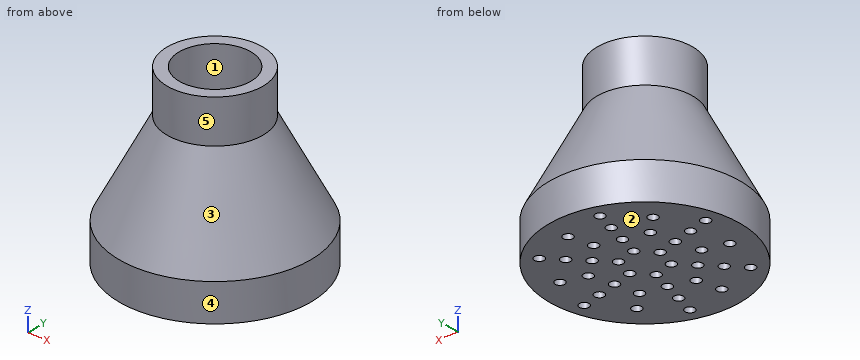
```python
from build123d import *

# Parameters (mm, degrees)
F0_R     = 25.4
F1_DEPTH = 31.75
F4_T     = -2.54
F5_R     = 12.7
F5_R_2   = 9.525
F6_DEPTH = 11.43
F7_R     = 25.4
F7_R_2   = 1.27
F8_DEPTH = 2.54


with BuildPart() as f1:
    # F0 (on Top) → F1 (new body)
    with BuildSketch(Plane.XY):
        Circle(F0_R)
    extrude(amount=F1_DEPTH)

    # F2 (on Right) → F3 (revolve, cut)
    with BuildSketch(Plane.YZ):
        Polygon((-29.21, 31.75), (-29.21, 0), (-12.7, 31.75), align=None)
    revolve(axis=Axis((0, 0, 15.875), (0, 0, -1)), mode=Mode.SUBTRACT)

    # F4
    f4_openings = [f1.faces().sort_by_distance(p)[0] for p in [
        (0, 0, 0),
        (0, 0, 31.75),
    ]]
    offset(amount=F4_T, openings=f4_openings)

    # F5 (on face) → F6 (join)
    with BuildSketch(Plane.XY.offset(31.75)):
        Circle(F5_R)
        Circle(F5_R_2, mode=Mode.SUBTRACT)
    extrude(amount=F6_DEPTH)

    # F7 (on face) → F8 (join)
    with BuildSketch(Plane(origin=(0, 0, 0), x_dir=(1, 0, 0), z_dir=(0, 0, -1))):
        Circle(F7_R)
        with Locations((-13.470384, -13.470384)):
            Circle(F7_R_2, mode=Mode.SUBTRACT)
        with Locations((-5.578226, -20.818224)):
            Circle(F7_R_2, mode=Mode.SUBTRACT)
        with Locations((-4.18367, -15.613668)):
            Circle(F7_R_2, mode=Mode.SUBTRACT)
        with Locations((-20.818224, -5.578226)):
            Circle(F7_R_2, mode=Mode.SUBTRACT)
        with Locations((-15.613668, -4.18367)):
            Circle(F7_R_2, mode=Mode.SUBTRACT)
        with Locations((-8.980256, -8.980256)):
            Circle(F7_R_2, mode=Mode.SUBTRACT)
        with Locations((-2.789113, -10.409112)):
            Circle(F7_R_2, mode=Mode.SUBTRACT)
        with Locations((-10.409112, -2.789113)):
            Circle(F7_R_2, mode=Mode.SUBTRACT)
        with Locations((-1.394557, -5.204557)):
            Circle(F7_R_2, mode=Mode.SUBTRACT)
        with Locations((-5.204557, -1.394557)):
            Circle(F7_R_2, mode=Mode.SUBTRACT)
        with Locations((4.930503, -18.400887)):
            Circle(F7_R_2, mode=Mode.SUBTRACT)
        with Locations((15.239998, -15.239998)):
            Circle(F7_R_2, mode=Mode.SUBTRACT)
        with Locations((3.287002, -12.267258)):
            Circle(F7_R_2, mode=Mode.SUBTRACT)
        with Locations((11.429998, -11.429998)):
            Circle(F7_R_2, mode=Mode.SUBTRACT)
        with Locations((7.619999, -7.619999)):
            Circle(F7_R_2, mode=Mode.SUBTRACT)
        with Locations((3.81, -3.81)):
            Circle(F7_R_2, mode=Mode.SUBTRACT)
        with Locations((12.267258, -3.287002)):
            Circle(F7_R_2, mode=Mode.SUBTRACT)
        with Locations((18.400887, -4.930503)):
            Circle(F7_R_2, mode=Mode.SUBTRACT)
        with Locations((-18.400887, 4.930503)):
            Circle(F7_R_2, mode=Mode.SUBTRACT)
        with Locations((-12.267258, 3.287002)):
            Circle(F7_R_2, mode=Mode.SUBTRACT)
        with Locations((-3.81, 3.81)):
            Circle(F7_R_2, mode=Mode.SUBTRACT)
        with Locations((-7.619999, 7.619999)):
            Circle(F7_R_2, mode=Mode.SUBTRACT)
        with Locations((-11.429998, 11.429998)):
            Circle(F7_R_2, mode=Mode.SUBTRACT)
        with Locations((-3.287002, 12.267258)):
            Circle(F7_R_2, mode=Mode.SUBTRACT)
        with Locations((-15.239998, 15.239998)):
            Circle(F7_R_2, mode=Mode.SUBTRACT)
        with Locations((-4.930503, 18.400887)):
            Circle(F7_R_2, mode=Mode.SUBTRACT)
        with Locations((5.204557, 1.394557)):
            Circle(F7_R_2, mode=Mode.SUBTRACT)
        with Locations((1.394557, 5.204557)):
            Circle(F7_R_2, mode=Mode.SUBTRACT)
        with Locations((10.409112, 2.789113)):
            Circle(F7_R_2, mode=Mode.SUBTRACT)
        with Locations((2.789113, 10.409112)):
            Circle(F7_R_2, mode=Mode.SUBTRACT)
        with Locations((8.980256, 8.980256)):
            Circle(F7_R_2, mode=Mode.SUBTRACT)
        with Locations((15.613668, 4.18367)):
            Circle(F7_R_2, mode=Mode.SUBTRACT)
        with Locations((20.818224, 5.578226)):
            Circle(F7_R_2, mode=Mode.SUBTRACT)
        with Locations((4.18367, 15.613668)):
            Circle(F7_R_2, mode=Mode.SUBTRACT)
        with Locations((5.578226, 20.818224)):
            Circle(F7_R_2, mode=Mode.SUBTRACT)
        with Locations((13.470384, 13.470384)):
            Circle(F7_R_2, mode=Mode.SUBTRACT)
    extrude(amount=F8_DEPTH)


solid = f1.part
```
The model under review builds one solid part; all positions refer to its coordinate system, in mm. Face numbers are marked on the shaded views. A direction names the side the tool comes from. Round coordinates to 2 decimals unless told otherwise and drop trailing zeros. Loops run counter-clockwise (first coordinate to the right, second up) from the corner with the lowest first, then second, coordinate; pieces in that order, holes last.
Item 1: Clearance check with flat-ended pins moving along their axes: pin 1 Ø4 at (x, y) = (-11.43, -11.43) entering from +Z; pin 2 Ø5 at (x, z) = (-11, 13) entering from +Y; pin 3 Ø2 at (x, y) = (4.18, -15.61) entering from -Z; pin 4 Ø2 at (x, y) = (-1.39, 5.2) entering from +Z. State where each tip first meets the part, or that it passes through.
Determined:
pin 1: stops at z = 28.93
pin 2: stops at y = 21.48
pin 3: stops at z = 17.67
pin 4: passes through
Item 2: For the marked faces 4 and 5, list the 3-axis set-ups (+Z, -Z, +X, -X, +Y, -Y) from which the entire face can be reached by the end or side of a thin tool; tool diameter is ignored.
Determined:
face 4: +Z, -Z
face 5: +Z
Item 3: Take a section at A-A (z = 19.5). Write out the cut boundary in (x, y).
Determined:
outline: circle Ø38.14 at (0, 0); hole circle Ø32.41 at (0, 0)
Item 4: Mouldability with a two-part tool opening along Z and no side actions: class the marked faces 1, 2 and 3 as released by +Z, released by -Z, zero draft, split by the parting line, or undercut.
Determined:
face 1: zero draft
face 2: released by -Z
face 3: released by +Z
Item 5: Take a section at B-B (z = 14). Write out the cut boundary in (x, y), then the cut area to 3 significant figures.
Determined:
outline: circle Ø43.86 at (0, 0); hole circle Ø38.13 at (0, 0)
area: 369 mm2
Item 6: For line 1 (X direction, y = -16.5, z = 9); line 2 (Y direction, x = -13, z = 17); line 3 (Y direction, x = 15, z = 2.5), list the stretches that pass through material, from the lowest coordinate up.
Determined:
line 1: x = -18.15 to -14.04, 14.04 to 18.15
line 2: y = -15.68 to -11.73, 11.73 to 15.68
line 3: y = -20.5 to -17.25, 17.25 to 20.5
